Input: part model. Units: mm. Frame: model coordinates. Face numbers are marked on the shaded views. A direction names the side the tool comes from. Give positions to 0.01 mm unless a question says otherwise; leave off trailing zeros. Write each loop counter-clockwise with the first axis right and the second up, starting at its lowest first coordinate (ties: lowest second). Pieces come first, ordered by that corner, then holes. Notation, with made-up numbers: (-33, -32.5) - (-18, -32.5) arc R27 cw to (-18, 1.5) - close; hole circle Ø2 at (49.25, -20.5). An arc over 180 degrees is marked (long way). Use a Markdown table: item, result. Add a question column.
1. Material intervals for probe 1 along X at (y, z) = (6, 14.25); probe 2 along X at (y, z) = (-7, 17.5), sorted ascending.
2. Pin query (flat end, axial travel): pin 1 (5 mm diameter, centred on x = -3.5, y = -9, fed in from +Z); pin 2 (4 mm diameter, centred on y = -0.5, z = 11, fed in from -X). Return the tip coordinate at first contact, or that it passes through.
3. Set-up query: the marked faces 5 and 6. Return all of +Z, -Z, +X, -X, +Y, -Y with unobstructed straight access to the full face (end or side cutting, diameter ignored); none if empty.
4. Section query C-C, the plane x = -6.5. Return loops of the section in (y, z), plus the area to 3 significant figures.
5. Section query D-D, the plane x = -3.5. Return loops of the section in (y, z), plus the area to 3 significant figures.
6. Section query B-B, the plane x = 2. Return loops of the section in (y, z), plus the area to 3 significant figures.
7. Section query A-A, the plane y = 9. Return loops of the section in (x, z), plus the area to 3 significant figures.
8. Mould query, pull axis Y, two halves, no side actions, for the marked faces 1, 2, 3 and 4. Classes: released by +Y, released by -Y, zero draft, split by the parting line, or undercut.
```python
from build123d import *

# Parameters (mm, degrees)
F1_DEPTH = 25.4
F2_R     = 5.08
F3_R     = 0.762


with BuildPart() as f1:
    # F0 (on Top) → F1 (new body)
    with BuildSketch(Plane.XY):
        Polygon((-11.2631590206, 12.7), (-9.2311590206, 10.668), (-4.2022368871, 10.668), (-4.2022368871, 12.7), align=None)
        Polygon((-12.7, 11.2631590206), (-10.668, 9.2311590206), (-10.668, 10.668), (-9.2311590206, 10.668), (-11.2631590206, 12.7), (-12.7, 12.7), align=None)
        Polygon((-10.668, 3.302), (-10.668, 9.2311590206), (-12.7, 11.2631590206), (-12.7, 3.302), align=None)
        Polygon((-12.7, -3.302), (-12.7, -11.2631590206), (-10.668, -9.2311590206), (-10.668, -3.302), align=None)
        Polygon((-12.7, -12.7), (-11.2631590206, -12.7), (-9.2311590206, -10.668), (-10.668, -10.668), (-10.668, -9.2311590206), (-12.7, -11.2631590206), align=None)
        Polygon((-11.2631590206, -12.7), (-4.2022368871, -12.7), (-4.2022368871, -10.668), (-9.2311590206, -10.668), align=None)
        Polygon((4.2022368871, -12.7), (11.2631590206, -12.7), (9.2311590206, -10.668), (4.2022368871, -10.668), align=None)
        Polygon((11.2631590206, -12.7), (12.7, -12.7), (12.7, -11.2631590206), (10.668, -9.2311590206), (10.668, -10.668), (9.2311590206, -10.668), align=None)
        Polygon((10.668, -9.2311590206), (12.7, -11.2631590206), (12.7, -3.302), (10.668, -3.302), align=None)
        Polygon((10.668, 3.302), (12.7, 3.302), (12.7, 11.2631590206), (10.668, 9.2311590206), align=None)
        Polygon((10.668, 9.2311590206), (12.7, 11.2631590206), (12.7, 12.7), (11.2631590206, 12.7), (9.2311590206, 10.668), (10.668, 10.668), align=None)
        Polygon((9.2311590206, 10.668), (11.2631590206, 12.7), (4.2022368871, 12.7), (4.2022368871, 10.668), align=None)
        with BuildLine():
            Line((-10.668, 9.2311590206), (-3.7321628684, 2.295321889))
            ThreePointArc((-3.7321628684, 2.295321889), (-3.0981883618, 3.0981883618), (-2.295321889, 3.7321628684))
            Line((-2.295321889, 3.7321628684), (-9.2311590206, 10.668))
            Line((-9.2311590206, 10.668), (-10.668, 10.668))
            Line((-10.668, 10.668), (-10.668, 9.2311590206))
        make_face()
        with BuildLine():
            Line((3.7321628684, 2.295321889), (10.668, 9.2311590206))
            Line((10.668, 9.2311590206), (10.668, 10.668))
            Line((10.668, 10.668), (9.2311590206, 10.668))
            Line((9.2311590206, 10.668), (2.295321889, 3.7321628684))
            ThreePointArc((2.295321889, 3.7321628684), (3.0981883618, 3.0981883618), (3.7321628684, 2.295321889))
        make_face()
        with BuildLine():
            Line((-9.2311590206, -10.668), (-2.295321889, -3.7321628684))
            ThreePointArc((-2.295321889, -3.7321628684), (-3.0981883618, -3.0981883618), (-3.7321628684, -2.295321889))
            Line((-3.7321628684, -2.295321889), (-10.668, -9.2311590206))
            Line((-10.668, -9.2311590206), (-10.668, -10.668))
            Line((-10.668, -10.668), (-9.2311590206, -10.668))
        make_face()
        with BuildLine():
            Line((2.295321889, -3.7321628684), (9.2311590206, -10.668))
            Line((9.2311590206, -10.668), (10.668, -10.668))
            Line((10.668, -10.668), (10.668, -9.2311590206))
            Line((10.668, -9.2311590206), (3.7321628684, -2.295321889))
            ThreePointArc((3.7321628684, -2.295321889), (3.0981883618, -3.0981883618), (2.295321889, -3.7321628684))
        make_face()
        with BuildLine():
            Line((0.9276876477, 2.3645286271), (2.295321889, 3.7321628684))
            ThreePointArc((2.295321889, 3.7321628684), (0, 4.3815), (-2.295321889, 3.7321628684))
            Line((-2.295321889, 3.7321628684), (-0.9276876477, 2.3645286271))
            ThreePointArc((-0.9276876477, 2.3645286271), (0, 2.54), (0.9276876477, 2.3645286271))
        make_face()
        with BuildLine():
            ThreePointArc((-2.295321889, 3.7321628684), (-3.0981883618, 3.0981883618), (-3.7321628684, 2.295321889))
            Line((-3.7321628684, 2.295321889), (-2.3645286271, 0.9276876477))
            ThreePointArc((-2.3645286271, 0.9276876477), (-1.7960512242, 1.7960512242), (-0.9276876477, 2.3645286271))
            Line((-0.9276876477, 2.3645286271), (-2.295321889, 3.7321628684))
        make_face()
        with BuildLine():
            ThreePointArc((-3.7321628684, 2.295321889), (-4.3815, 0), (-3.7321628684, -2.295321889))
            Line((-3.7321628684, -2.295321889), (-2.3645286271, -0.9276876477))
            ThreePointArc((-2.3645286271, -0.9276876477), (-2.54, 0), (-2.3645286271, 0.9276876477))
            Line((-2.3645286271, 0.9276876477), (-3.7321628684, 2.295321889))
        make_face()
        with BuildLine():
            ThreePointArc((-3.7321628684, -2.295321889), (-3.0981883618, -3.0981883618), (-2.295321889, -3.7321628684))
            Line((-2.295321889, -3.7321628684), (-0.9276876477, -2.3645286271))
            ThreePointArc((-0.9276876477, -2.3645286271), (-1.7960512242, -1.7960512242), (-2.3645286271, -0.9276876477))
            Line((-2.3645286271, -0.9276876477), (-3.7321628684, -2.295321889))
        make_face()
        with BuildLine():
            ThreePointArc((-2.295321889, -3.7321628684), (0, -4.3815), (2.295321889, -3.7321628684))
            Line((2.295321889, -3.7321628684), (0.9276876477, -2.3645286271))
            ThreePointArc((0.9276876477, -2.3645286271), (0, -2.54), (-0.9276876477, -2.3645286271))
            Line((-0.9276876477, -2.3645286271), (-2.295321889, -3.7321628684))
        make_face()
        with BuildLine():
            Line((2.3645286271, 0.9276876477), (3.7321628684, 2.295321889))
            ThreePointArc((3.7321628684, 2.295321889), (3.0981883618, 3.0981883618), (2.295321889, 3.7321628684))
            Line((2.295321889, 3.7321628684), (0.9276876477, 2.3645286271))
            ThreePointArc((0.9276876477, 2.3645286271), (1.7960512242, 1.7960512242), (2.3645286271, 0.9276876477))
        make_face()
        with BuildLine():
            Line((2.3645286271, -0.9276876477), (3.7321628684, -2.295321889))
            ThreePointArc((3.7321628684, -2.295321889), (4.2160416185, -1.1927008515), (4.3815, 0))
            ThreePointArc((4.3815, 0), (4.2160416185, 1.1927008515), (3.7321628684, 2.295321889))
            Line((3.7321628684, 2.295321889), (2.3645286271, 0.9276876477))
            ThreePointArc((2.3645286271, 0.9276876477), (2.4957466531, 0.4720684734), (2.54, 0))
            ThreePointArc((2.54, 0), (2.4957466531, -0.4720684734), (2.3645286271, -0.9276876477))
        make_face()
        with BuildLine():
            Line((0.9276876477, -2.3645286271), (2.295321889, -3.7321628684))
            ThreePointArc((2.295321889, -3.7321628684), (3.0981883618, -3.0981883618), (3.7321628684, -2.295321889))
            Line((3.7321628684, -2.295321889), (2.3645286271, -0.9276876477))
            ThreePointArc((2.3645286271, -0.9276876477), (1.7960512242, -1.7960512242), (0.9276876477, -2.3645286271))
        make_face()
    extrude(amount=F1_DEPTH)

    # F2
    f2_edges = [f1.edges().sort_by_distance(p)[0] for p in [
        (-3.732163, 2.295322, 12.7),
        (-3.732163, -2.295322, 12.7),
        (-2.295322, 3.732163, 12.7),
        (2.295322, 3.732163, 12.7),
        (-2.295322, -3.732163, 12.7),
        (2.295322, -3.732163, 12.7),
        (3.732163, -2.295322, 12.7),
        (3.732163, 2.295322, 12.7),
    ]]
    fillet(f2_edges, radius=F2_R)

    # F3
    f3_edges = [f1.edges().sort_by_distance(p)[0] for p in [
        (9.231159, 10.668, 12.7),
        (10.668, 9.231159, 12.7),
        (-9.231159, 10.668, 12.7),
        (-10.668, 9.231159, 12.7),
        (10.668, -9.231159, 12.7),
        (9.231159, -10.668, 12.7),
        (-9.231159, -10.668, 12.7),
        (-10.668, -9.231159, 12.7),
        (-12.7, 12.7, 12.7),
        (12.7, 12.7, 12.7),
        (12.7, -12.7, 12.7),
        (-12.7, -12.7, 12.7),
        (12.7, 3.302, 12.7),
        (10.668, 3.302, 12.7),
        (4.202237, 10.668, 12.7),
        (4.202237, 12.7, 12.7),
        (-4.202237, 12.7, 12.7),
        (-4.202237, 10.668, 12.7),
        (-10.668, 3.302, 12.7),
        (-12.7, 3.302, 12.7),
        (-10.668, -3.302, 12.7),
        (-12.7, -3.302, 12.7),
        (4.202237, -10.668, 12.7),
        (4.202237, -12.7, 12.7),
        (10.668, -3.302, 12.7),
        (12.7, -3.302, 12.7),
        (-4.202237, -12.7, 12.7),
        (-4.202237, -10.668, 12.7),
    ]]
    fillet(f3_edges, radius=F3_R)


solid = f1.part
```
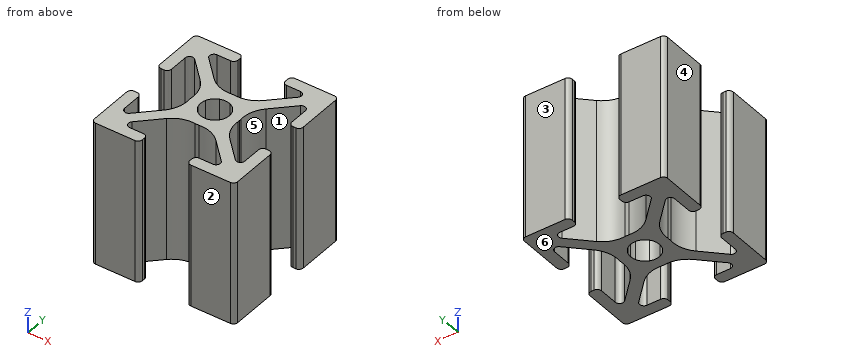
Result sheet:
| question | item | result |
|---|---|---|
| 1 | probe 1 | x = -12.7 to -10.67, -7.44 to -4.56, 4.56 to 7.44, 10.67 to 12.7 |
| 1 | probe 2 | x = -12.7 to -10.67, -8.44 to -5.56, 5.56 to 8.44, 10.67 to 12.7 |
| 2 | pin 1 | stops at z = 25.4 |
| 2 | pin 2 | stops at x = -4.64 |
| 3 | face 5 | +Z, -Z |
| 3 | face 6 | -Z, +X, -X, +Y, -Y |
| 4 | outline | (-12.7, 0) - (-10.67, 0) - (-10.67, 25.4) - (-12.7, 25.4) - close; (-7.94, 0) - (-5.06, 0) - (-5.06, 25.4) - (-7.94, 25.4) - close; (5.06, 0) - (7.94, 0) - (7.94, 25.4) - (5.06, 25.4) - close; (10.67, 0) - (12.7, 0) - (12.7, 25.4) - (10.67, 25.4) - close |
| 4 | area | 249 mm² |
| 5 | outline | (-5.12, 0) - (5.12, 0) - (5.12, 25.4) - (-5.12, 25.4) - close |
| 5 | area | 260 mm² |
| 6 | outline | (-4.49, 0) - (-1.57, 0) - (-1.57, 25.4) - (-4.49, 25.4) - close; (1.57, 0) - (4.49, 0) - (4.49, 25.4) - (1.57, 25.4) - close |
| 6 | area | 149 mm² |
| 7 | outline | (-12.7, 0) - (-7.56, 0) - (-7.56, 25.4) - (-12.7, 25.4) - close; (7.56, 0) - (12.7, 0) - (12.7, 25.4) - (7.56, 25.4) - close |
| 7 | area | 261 mm² |
| 8 | face 1 | undercut |
| 8 | face 2 | released by -Y |
| 8 | face 3 | released by +Y |
| 8 | face 4 | zero draft |
